Here's how the part is built. I have some questions about the finished solid (model axes, mm). Face numbers are marked on the shaded views. Give positions to 0.01 mm unless a question says otherwise; leave off trailing zeros. Write each loop counter-clockwise with the first axis right and the second up, starting at its lowest first coordinate (ties: lowest second). Pieces come first, ordered by that corner, then holes. Notation, with made-up numbers: M 2.25,54 L 49.25,54 A25 ccw 49.25,91 Z; hole C 0,87.5 d5. An arc over 180 degrees is marked long. Answer as CSV lines item,"result". Start each with the question number.
Q1. If I drill on line 1 along Y through (x, z) = (0.55, 0); line 2 along Y through (x, z) = (0.1, 0); line 3 along X through (y, z) = (2, -1), over which ranges is the centre line in solid material (lowest first)?
Q2. Suppose I cut it at C-C (x = 0.55). Write out the boundary of the cut face in (y, z), then the cut area to 3 significant figures.
Q3. Suppose I cut it at D-D (z = 2.5). Write out the boundary of the cut face in (x, y), then the cut area to 3 significant figures.
Q4. For pin 1 (1 mm diameter, centred on y = -3, z = -0.5, fed in from -X), with a flat end and sliding along its axis, tell me the tip position at first contact or that it passes through.
Q5. Suppose I cut it at A-A (z = 0). Write out the boundary of the cut face in (x, y), then the cut area to 3 significant figures.
Q6. Thinking about a two-plate mould opening in Z: for the marked faces 1, 2 and 3, which applies, +Z half, -Z half, draft (parallel to the pull), parting line (faces both ways), or undercut?
```python
from build123d import *

# Parameters (mm, degrees)
SKETCH_1_R          = 5
EXTRUDE_301_DEPTH   = 2
SKETCH_9_R          = 4.442422665
CUT_EXTRUDE_2_DEPTH = 0.2
SKETCH_10_R         = 0.75956549
CUT_EXTRUDE_3_DEPTH = 0.6
SKETCH_11_R         = 0.278093265
CUT_EXTRUDE_4_DEPTH = 0.6


with BuildPart() as part:
    # 草图1 → Extrude 301 (new body)
    with BuildSketch(Plane(origin=(0, 0, 0), x_dir=(0, 0, -1), z_dir=(1, 0, 0))):
        Circle(SKETCH_1_R)
    extrude(amount=EXTRUDE_301_DEPTH)

    # 草图9 → 切除-拉伸2 (cut)
    with BuildSketch(Plane.ZY):
        Circle(SKETCH_9_R)
    extrude(amount=-CUT_EXTRUDE_2_DEPTH, mode=Mode.SUBTRACT)

    # 草图10 → 切除-拉伸3 (cut)
    with BuildSketch(Plane.ZY.offset(-0.2)):
        Circle(SKETCH_10_R)
    extrude(amount=-CUT_EXTRUDE_3_DEPTH, mode=Mode.SUBTRACT)

    # 草图11 → 切除-拉伸4 (cut)
    with BuildSketch(Plane.ZY.offset(-0.8)):
        Circle(SKETCH_11_R)
    extrude(amount=-CUT_EXTRUDE_4_DEPTH, mode=Mode.SUBTRACT)


solid = part.part
```
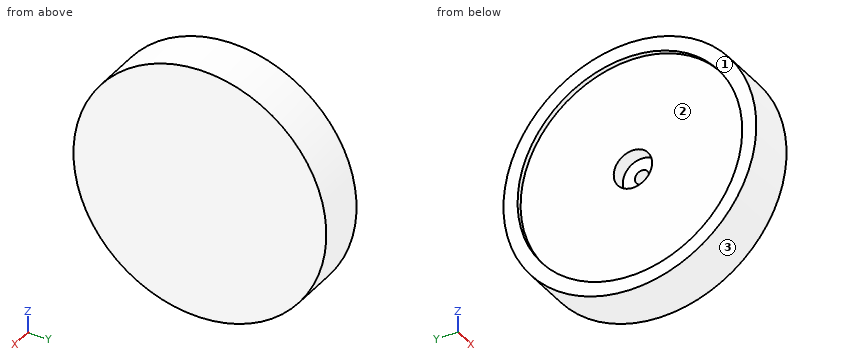
Resolved:
1,line 1,"-5 to -0.76, 0.76 to 5"
1,line 2,"-5 to -4.44, 4.44 to 5"
1,line 3,"0.2 to 2"
2,outline,"C 0,0 d10; hole C 0,0 d1.52"
2,area,"76.7 mm^2"
3,outline,"M 0,-4.33 L 2,-4.33 L 2,4.33 L 0,4.33 L 0,3.67 L 0.2,3.67 L 0.2,-3.67 L 0,-3.67 Z"
3,area,"15.9 mm^2"
4,pin 1,"x = 0.2"
5,outline,"M 0,-5 L 2,-5 L 2,5 L 0,5 L 0,4.44 L 0.2,4.44 L 0.2,0.76 L 0.8,0.76 L 0.8,0.28 L 1.4,0.28 L 1.4,-0.28 L 0.8,-0.28 L 0.8,-0.76 L 0.2,-0.76 L 0.2,-4.44 L 0,-4.44 Z"
5,area,"17.0 mm^2"
6,face 1,"draft"
6,face 2,"undercut"
6,face 3,"parting line"
